```python
from build123d import *

# Parameters (mm, degrees)
SKETCH_1_W          = 42
SKETCH_1_H          = 20
EXTRUDE_1_DEPTH     = 60
SKETCH_3_W          = 30
SKETCH_3_H          = 54
CUT_EXTRUDE_1_DEPTH = 67.640828326
FILLET_1_R          = 6
SKETCH_4_R          = 4
CUT_EXTRUDE_2_DEPTH = 74.91887445


with BuildPart() as part:
    # 草图1 → 凸台-拉伸1 (new body)
    with BuildSketch(Plane.XY):
        Rectangle(SKETCH_1_W, SKETCH_1_H)
    extrude(amount=-EXTRUDE_1_DEPTH)

    # 草图3 → 切除-拉伸1 (cut, through all)
    with BuildSketch(Plane.XZ.offset(10)):
        with Locations((0, -33)):
            Rectangle(SKETCH_3_W, SKETCH_3_H)
    extrude(amount=-CUT_EXTRUDE_1_DEPTH, mode=Mode.SUBTRACT)

    # 圆角1
    fillet_1_edges = [part.edges().sort_by_distance(p)[0] for p in [
        (18, 10, -60),
        (-18, 10, -60),
        (18, -10, -60),
        (-15, 0, -6),
        (15, 0, -6),
        (21, 0, 0),
        (-21, 0, 0),
        (-18, -10, -60),
    ]]
    fillet(fillet_1_edges, radius=FILLET_1_R)

    # 草图4 → 切除-拉伸2 (cut, through all)
    with BuildSketch(Plane(origin=(21, 0, 0), x_dir=(0, 0, -1), z_dir=(1, 0, 0))):
        with Locations((50, 0)):
            Circle(SKETCH_4_R)
    extrude(amount=-CUT_EXTRUDE_2_DEPTH, mode=Mode.SUBTRACT)


solid = part.part
```
Input: part model. Units: mm. Frame: model coordinates. A direction names the side the tool comes from. Give positions to 0.01 mm unless a question says otherwise; leave off trailing zeros. Order: outer loops, then holes, each group sorted by start corner. A loop starts at its lowest first (then second) coordinate and runs counter-clockwise, first axis right, second up.
1. Section B-B on y = 0. Return the cut outline in (x, z).
Derived:
outline: (-21, -60) - (-15, -60) - (-15, -54) - (-21, -54) - close; (-21, -46) - (-15, -46) - (-15, -12) arc R6 cw to (-9, -6) - (9, -6) arc R6 cw to (15, -12) - (15, -46) - (21, -46) - (21, -6) arc R6 ccw to (15, 0) - (-15, 0) arc R6 ccw to (-21, -6) - close; (15, -60) - (21, -60) - (21, -54) - (15, -54) - close
2. Section A-A on z = -50. Return the cut outline in (x, y).
Derived:
outline: (-21, -10) - (-15, -10) - (-15, -4) - (-21, -4) - close; (-21, 4) - (-15, 4) - (-15, 10) - (-21, 10) - close; (15, -10) - (21, -10) - (21, -4) - (15, -4) - close; (15, 4) - (21, 4) - (21, 10) - (15, 10) - close
3. Mould query, pull axis Y, two halves, no side actions, for faces 3 (the cylindrical face through (-17.958, -8.289, -58.196)), 4 (the cylindrical face through (-18, 0, -46)), 5 (the cylindrical face through (-19.289, 0.14, -1.804)). Classes: released by +Y, released by -Y, zero draft, split by the parting line, or undercut.
Derived:
face 3: released by -Y
face 4: undercut
face 5: zero draft
4. Material intervals for L1, parallel to X at y = -1, z = -26; L2, parallel to Y at x = -19, z = -50; L3, parallel to Z at x = 17.5, y = 3.25, sorted ascending.
Derived:
L1: x = -21 to -15, 15 to 21
L2: y = -10 to -4, 4 to 10
L3: z = -60 to -52.33, -47.67 to -0.55
5. Section C-C on z = -33.5. Return the cut outline in (x, y), and give its area (3 significant figures).
Derived:
outline: (-21, -10) - (-15, -10) - (-15, 10) - (-21, 10) - close; (15, -10) - (21, -10) - (21, 10) - (15, 10) - close
area: 240 mm2
6. Section D-D on x = 17. Return the cut outline in (y, z).
Derived:
outline: (-10, -54) arc R6 ccw to (-4, -60) - (4, -60) arc R6 ccw to (10, -54) - (10, -0.34) - (-10, -0.34) - close; hole circle Ø8 at (0, -50)
7. Pin query (flat end, axial travel): pin 1 (12 mm diameter, centred on x = 8, z = -25, fed in from -Y). Return the tip coordinate at first contact, or that it passes through.
Derived:
pin 1: passes through
8. Reachability of faces 1 (the cylindrical face through (-13.196, 0.14, -7.711)), 2 (the flat face through (0, 0, 0)) from +Z, -Z, +X, -X, +Y, -Y: full face, straight path, thin tool, end or side. Return the list, or none.
Derived:
face 1: -Z, +Y, -Y
face 2: +Z, +X, -X, +Y, -Y
